Check sheet for the modelled part. Datum: model origin and axes. Units: mm. A direction names the side the tool comes from. Coordinates: 2 decimals unless noted, no trailing zeros. Loops run counter-clockwise (first coordinate to the right, second up) from the corner with the lowest first, then second, coordinate; pieces in that order, holes last.
from build123d import *

# Parameters (mm, degrees)
SKETCH1_R               = 3.65
SKETCH1_W               = 26.6
SKETCH1_H               = 32.3
BOSS_EXTRUDE1_DEPTH     = 8
SKETCH2_W               = 3
SKETCH2_H               = 0.7
BOSS_EXTRUDE2_DEPTH     = 1.2
SKETCH3_W               = 3
SKETCH3_H               = 0.7
BOSS_EXTRUDE3_DEPTH     = 1.2
CHAMFER1_SIZE           = 1.2
CUT_EXTRUDE1_DEPTH      = 85.642077968
CUT_EXTRUDE1_DEPTH_BACK = 85.642077968
SKETCH4_W               = 48.801078557
SKETCH4_H               = 1.4
SKETCH4_W_2             = 10.59579159
SKETCH4_W_3             = 46.838011079
BOSS_EXTRUDE4_START     = -5.4
SKETCH5_W               = 13
SKETCH5_H               = 1.2
SKETCH5_W_2             = 1.2
SKETCH5_H_2             = 13
BOSS_EXTRUDE4_DEPTH     = 2.8
BOSS_EXTRUDE5_REACH     = 77.99
SKETCH7_W               = 1.2
SKETCH7_H               = 1.202104206
SKETCH7_H_2             = 1.201731925
BOSS_EXTRUDE6_DEPTH     = 7
SKETCH8_W               = 1.202104206
SKETCH8_H               = 1.3
SKETCH8_W_2             = 1.201731925
BOSS_EXTRUDE7_DEPTH     = 26.6
SKETCH9_W               = 1.2
SKETCH9_H               = 1.3
BOSS_EXTRUDE8_DEPTH     = 11.797895795


with BuildPart() as part:
    # Sketch1 → Boss-Extrude1 (new body)
    with BuildSketch(Plane(origin=(0, 0, 0), x_dir=(1, 0, 0), z_dir=(0, 1, 0))):
        with BuildLine():
            Line((-7.021942446, 23.451798561), (-15.021942446, 23.451798561))
            Line((-15.021942446, 23.451798561), (-15.021942446, 12.601798561))
            Line((-15.021942446, 12.601798561), (-45.721942446, 10.951798561))
            ThreePointArc((-45.721942446, 10.951798561), (-50.571942446, 6.101798561), (-45.721942446, 1.251798561))
            Line((-45.721942446, 1.251798561), (-15.021942446, -0.398201439))
            Line((-15.021942446, -0.398201439), (-15.021942446, -11.248201439))
            Line((-15.021942446, -11.248201439), (-7.021942446, -11.248201439))
            Line((-7.021942446, -11.248201439), (-5.371942446, -39.098201439))
            ThreePointArc((-5.371942446, -39.098201439), (-0.521942446, -43.948201439), (4.328057554, -39.098201439))
            Line((4.328057554, -39.098201439), (5.978057554, -11.248201439))
            Line((5.978057554, -11.248201439), (13.978057554, -11.248201439))
            Line((13.978057554, -11.248201439), (13.978057554, -0.398201439))
            Line((13.978057554, -0.398201439), (44.678057554, 1.251798561))
            ThreePointArc((44.678057554, 1.251798561), (49.528057554, 6.101798561), (44.678057554, 10.951798561))
            Line((44.678057554, 10.951798561), (13.978057554, 12.601798561))
            Line((13.978057554, 12.601798561), (13.978057554, 23.451798561))
            Line((13.978057554, 23.451798561), (5.978057554, 23.451798561))
            Line((5.978057554, 23.451798561), (4.328057554, 51.301798561))
            ThreePointArc((4.328057554, 51.301798561), (-0.521942446, 56.151798561), (-5.371942446, 51.301798561))
            Line((-5.371942446, 51.301798561), (-7.021942446, 23.451798561))
        make_face()
        with Locations(Location((-0.521942446, -39.098201439, 0), (0, 0, 270))):
            Circle(SKETCH1_R, mode=Mode.SUBTRACT)
        with BuildLine():
            Line((4.775953349, -11.248201439), (3.302651218, -36.115755579))
            ThreePointArc((3.302651218, -36.115755579), (-0.521942446, -34.248201439), (-4.34653611, -36.115755579))
            Line((-4.34653611, -36.115755579), (-5.819838241, -11.248201439))
            Line((-5.819838241, -11.248201439), (4.775953349, -11.248201439))
        make_face(mode=Mode.SUBTRACT)
        with Locations(Location((-45.721942446, 6.101798561, 0), (0, 0, 270))):
            Circle(SKETCH1_R, mode=Mode.SUBTRACT)
        with BuildLine():
            Line((-42.720356894, 9.911389638), (-15.021942446, 11.400066636))
            Line((-15.021942446, 11.400066636), (-15.021942446, 0.803530486))
            Line((-15.021942446, 0.803530486), (-42.720356894, 2.292207484))
            ThreePointArc((-42.720356894, 2.292207484), (-40.871942446, 6.101798561), (-42.720356894, 9.911389638))
        make_face(mode=Mode.SUBTRACT)
        with Locations((-0.521942446, 6.101798561)):
            Rectangle(SKETCH1_W, SKETCH1_H, mode=Mode.SUBTRACT)
        with BuildLine():
            Line((-5.819838241, 23.451798561), (-4.34653611, 48.319352702))
            ThreePointArc((-4.34653611, 48.319352702), (-0.521942446, 46.451798561), (3.302651218, 48.319352702))
            Line((3.302651218, 48.319352702), (4.775953349, 23.451798561))
            Line((4.775953349, 23.451798561), (-5.819838241, 23.451798561))
        make_face(mode=Mode.SUBTRACT)
        with Locations(Location((-0.521942446, 51.301798561, 0), (0, 0, 270))):
            Circle(SKETCH1_R, mode=Mode.SUBTRACT)
        with BuildLine():
            Line((41.676472002, 2.292207484), (13.978057554, 0.803530486))
            Line((13.978057554, 0.803530486), (13.978057554, 11.400066636))
            Line((13.978057554, 11.400066636), (41.676472002, 9.911389638))
            ThreePointArc((41.676472002, 9.911389638), (39.828057554, 6.101798561), (41.676472002, 2.292207484))
        make_face(mode=Mode.SUBTRACT)
        with Locations(Location((44.678057554, 6.101798561, 0), (0, 0, 270))):
            Circle(SKETCH1_R, mode=Mode.SUBTRACT)
    extrude(amount=BOSS_EXTRUDE1_DEPTH)

    # Sketch2 → Boss-Extrude2 (add)
    with BuildSketch(Plane.XY.offset(-22.251798561)):
        with Locations((-2.021942446, 6.05)):
            Rectangle(SKETCH2_W, SKETCH2_H)
        with Locations((0.978057554, 6.05)):
            Rectangle(SKETCH2_W, SKETCH2_H)
    extrude(amount=BOSS_EXTRUDE2_DEPTH)

    # Sketch3 → Boss-Extrude3 (add)
    with BuildSketch(Plane(origin=(0, 0, 10.048201439), x_dir=(-1, 0, 0), z_dir=(0, 0, -1))):
        with Locations((-0.978057554, 6.05)):
            Rectangle(SKETCH3_W, SKETCH3_H)
        with Locations((2.021942446, 6.05)):
            Rectangle(SKETCH3_W, SKETCH3_H)
    extrude(amount=BOSS_EXTRUDE3_DEPTH)

    # Chamfer1
    chamfer1_edges = [part.edges().sort_by_distance(p)[0] for p in [
        (-0.521942446, 5.7, -22.251798561),
        (-0.521942446, 5.7, 10.048201439),
    ]]
    chamfer(chamfer1_edges, length=CHAMFER1_SIZE - 0.0001)  # a hair under: the kernel refuses the full size

    # Sketch4 → Cut-Extrude1 (cut, two sides: drawn at the far end of the back side and taken through both)
    with BuildSketch(Plane(origin=(0, 0, -23.451798561), x_dir=(-1, 0, 0), z_dir=(0, 0, -1)).offset(-CUT_EXTRUDE1_DEPTH_BACK)):
        with Locations((-29.176492628, 3.3)):
            Rectangle(SKETCH4_W, SKETCH4_H)
        with Locations((-29.176492628, 4.7)):
            Rectangle(SKETCH4_W, SKETCH4_H)
        with Locations((0.521942446, 4.7)):
            Rectangle(SKETCH4_W_2, SKETCH4_H)
        with Locations((0.521942446, 3.3)):
            Rectangle(SKETCH4_W_2, SKETCH4_H)
        with Locations((29.238843781, 3.3)):
            Rectangle(SKETCH4_W_3, SKETCH4_H)
        with Locations((29.238843781, 4.7)):
            Rectangle(SKETCH4_W_3, SKETCH4_H)
    extrude(amount=CUT_EXTRUDE1_DEPTH + CUT_EXTRUDE1_DEPTH_BACK, mode=Mode.SUBTRACT)


with BuildPart() as cut_extrude1_piece_1:
    # of the separate pieces the step leaves, piece 1, a body of its own (cut_extrude1_pieces)
    add(part.part.solids().sort_by_distance((-3.521942446, 6.4, 10.048201439))[0])



with BuildPart() as cut_extrude1_piece_2:
    # of the separate pieces the step leaves, piece 2, a body of its own (cut_extrude1_pieces)
    add(part.part.solids().sort_by_distance((12.778057554, 2.6, 10.048201439))[0])


with BuildPart() as cut_extrude1_piece_1_1:
    add(cut_extrude1_piece_1.part)

    add(cut_extrude1_piece_2.part)  # Boss-Extrude4 merges Cut-Extrude1 piece 2
    # Sketch5 → Boss-Extrude4 (add)
    with BuildSketch(Plane(origin=(0, 8, 0), x_dir=(1, 0, 0), z_dir=(0, 1, 0)).offset(BOSS_EXTRUDE4_START)):
        with Locations((-0.521942446, 22.851798561)):
            Rectangle(SKETCH5_W, SKETCH5_H)
        with Locations((-0.521942446, -10.648201439)):
            Rectangle(SKETCH5_W, SKETCH5_H)
        with Locations((-14.421942446, 6.101798561)):
            Rectangle(SKETCH5_W_2, SKETCH5_H_2)
        with Locations((13.378057554, 6.101798561)):
            Rectangle(SKETCH5_W_2, SKETCH5_H_2)
    extrude(amount=BOSS_EXTRUDE4_DEPTH)

    # Sketch6 → Boss-Extrude5 (add, up to next)
    with BuildSketch(Plane(origin=(0, 8, 0), x_dir=(1, 0, 0), z_dir=(0, 1, 0)), mode=Mode.PRIVATE) as boss_extrude5_sk1:
        with BuildLine():
            Line((-5.371942446, 51.301798561), (-4.171942446, 51.301798561))
            ThreePointArc((-4.171942446, 51.301798561), (-0.521942446, 54.951798561), (3.128057554, 51.301798561))
            Line((3.128057554, 51.301798561), (4.328057554, 51.301798561))
            ThreePointArc((4.328057554, 51.301798561), (-0.521942446, 56.151798561), (-5.371942446, 51.301798561))
        make_face()
    boss_extrude5_tool1 = extrude(boss_extrude5_sk1.sketch, amount=-BOSS_EXTRUDE5_REACH, mode=Mode.PRIVATE) - cut_extrude1_piece_1_1.part
    # Sketch6 → Boss-Extrude5 (add, up to next)
    with BuildSketch(Plane(origin=(0, 8, 0), x_dir=(1, 0, 0), z_dir=(0, 1, 0)), mode=Mode.PRIVATE) as boss_extrude5_sk2:
        with BuildLine():
            Line((3.128057554, -39.098201439), (4.328057554, -39.098201439))
            ThreePointArc((4.328057554, -39.098201439), (-0.521942446, -43.948201439), (-5.371942446, -39.098201439))
            Line((-5.371942446, -39.098201439), (-4.171942446, -39.098201439))
            ThreePointArc((-4.171942446, -39.098201439), (-0.521942446, -42.748201439), (3.128057554, -39.098201439))
        make_face()
    boss_extrude5_tool2 = extrude(boss_extrude5_sk2.sketch, amount=-BOSS_EXTRUDE5_REACH, mode=Mode.PRIVATE) - cut_extrude1_piece_1_1.part
    # Sketch6 → Boss-Extrude5 (add, up to next)
    with BuildSketch(Plane(origin=(0, 8, 0), x_dir=(1, 0, 0), z_dir=(0, 1, 0)), mode=Mode.PRIVATE) as boss_extrude5_sk3:
        with BuildLine():
            Line((44.678057554, 9.751798561), (44.678057554, 10.951798561))
            ThreePointArc((44.678057554, 10.951798561), (49.528057554, 6.101798561), (44.678057554, 1.251798561))
            Line((44.678057554, 1.251798561), (44.678057554, 2.451798561))
            ThreePointArc((44.678057554, 2.451798561), (48.328057554, 6.101798561), (44.678057554, 9.751798561))
        make_face()
    boss_extrude5_tool3 = extrude(boss_extrude5_sk3.sketch, amount=-BOSS_EXTRUDE5_REACH, mode=Mode.PRIVATE) - cut_extrude1_piece_1_1.part
    # Sketch6 → Boss-Extrude5 (add, up to next)
    with BuildSketch(Plane(origin=(0, 8, 0), x_dir=(1, 0, 0), z_dir=(0, 1, 0)), mode=Mode.PRIVATE) as boss_extrude5_sk4:
        with BuildLine():
            Line((-45.721942446, 1.251798561), (-45.721942446, 2.451798561))
            ThreePointArc((-45.721942446, 2.451798561), (-49.371942446, 6.101798561), (-45.721942446, 9.751798561))
            Line((-45.721942446, 9.751798561), (-45.721942446, 10.951798561))
            ThreePointArc((-45.721942446, 10.951798561), (-50.571942446, 6.101798561), (-45.721942446, 1.251798561))
        make_face()
    boss_extrude5_tool4 = extrude(boss_extrude5_sk4.sketch, amount=-BOSS_EXTRUDE5_REACH, mode=Mode.PRIVATE) - cut_extrude1_piece_1_1.part
    add(boss_extrude5_tool1.solids().sort_by_distance((-4.771942, 8, -51.410248))[0])
    add(boss_extrude5_tool2.solids().sort_by_distance((-0.521942, 8, 43.839752))[0])
    add(boss_extrude5_tool3.solids().sort_by_distance((44.786507, 8, -10.351799))[0])
    add(boss_extrude5_tool4.solids().sort_by_distance((-45.830392, 8, -10.351799))[0])

    # Sketch7 → Boss-Extrude6 (add)
    with BuildSketch(Plane.XZ):
        with Locations((-14.421942446, -0.202850664)):
            Rectangle(SKETCH7_W, SKETCH7_H)
        with Locations((-14.421942446, -12.000932599)):
            Rectangle(SKETCH7_W, SKETCH7_H_2)
        with Locations((13.378057554, -0.202850664)):
            Rectangle(SKETCH7_W, SKETCH7_H)
        with Locations((13.378057554, -12.000932599)):
            Rectangle(SKETCH7_W, SKETCH7_H_2)
    extrude(amount=BOSS_EXTRUDE6_DEPTH)

    # Sketch8 → Boss-Extrude7 (add)
    with BuildSketch(Plane(origin=(-13.821942446, 0, 0), x_dir=(0, 0, -1), z_dir=(1, 0, 0))):
        with Locations((0.202850664, -6.35)):
            Rectangle(SKETCH8_W, SKETCH8_H)
        with Locations((12.000932599, -6.35)):
            Rectangle(SKETCH8_W_2, SKETCH8_H)
    extrude(amount=BOSS_EXTRUDE7_DEPTH)

    # Sketch9 → Boss-Extrude8 (add)
    with BuildSketch(Plane(origin=(0, 0, -12.601798561), x_dir=(-1, 0, 0), z_dir=(0, 0, -1))):
        with Locations((-13.378057554, -6.35)):
            Rectangle(SKETCH9_W, SKETCH9_H)
        with Locations((14.421942446, -6.35)):
            Rectangle(SKETCH9_W, SKETCH9_H)
    extrude(amount=-BOSS_EXTRUDE8_DEPTH)


solid = cut_extrude1_piece_1_1.part
(1) Draft check along Z on faces 4 (the face through (-14, 5.4, -20)), 5 (the face through (4.05, 1.28, 23.51)), 6 (the face through (29.113, 6.682, -0.415)). Enter one of: pulls with the +Z half, pulls with the -Z half, needs draft (parallel to the pull), parting line crosses it, or undercut.
(2) Section check C-C, the plane y = -3. Enter the section's corners in (x, z).
(3) Section check B-B, the plane y = 4.25. Count the separate pieces of the cut face and the enclosed holes in it, plus the area to 3 significant figures.
(4) Gauge pin test, flat ends, axial feed: P1, Ø4, axis at y = 0, z = -29.5, coming from the +X side; P2, Ø1.3, axis at x = -14.5, y = 4.5, coming from the -Z side; P3, Ø1.3, axis at x = -5.5, z = -0.5, coming from the +Y side; P4, Ø3, axis at y = -2, z = 31, coming from the -X side. Record the tip position at first contact, or that the pin passes through.
(5) Scan lines: line 1 along X through (y, z) = (5.75, -22); line 2 along Z through (x, y) = (40.5, 6.25); line 3 along Y through (x, z) = (-5, -42). Record each from-to range of solid material in increasing order.
(6) Set-up check for faces 1 (the face through (30, 5.4, -1)), 2 (the face through (13, 5.4, -20)), 3 (the face through (10, 7, 11.248)): record each of +Z, -Z, +X, -X, +Y, -Y from which the full face is reachable in a straight line by a thin tool's end or side.
(7) Section check A-A, the plane z = -18. Enter the section's corners in (x, y), plus the area to 3 significant figures.
Determined:
1. face 4: needs draft
1. face 5: undercut
1. face 6: pulls with the +Z half
2. outline: (-15.02, -12.6) - (-13.82, -12.6) - (-13.82, -11.4) - (-15.02, -11.4) - close; (-15.02, -0.8) - (-13.82, -0.8) - (-13.82, 0.4) - (-15.02, 0.4) - close; (12.78, -12.6) - (13.98, -12.6) - (13.98, -11.4) - (12.78, -11.4) - close; (12.78, -0.8) - (13.98, -0.8) - (13.98, 0.4) - (12.78, 0.4) - close
3. separate pieces: 8
3. enclosed holes: 0
3. area: 126 mm2
4. P1: stops at x = 5.74
4. P2: stops at z = -12.6
4. P3: stops at y = -5.7
4. P4: passes through
5. line 1: x = -15.02 to -13.82, -3.52 to 2.48, 12.78 to 13.98
5. line 2: z = -11.18 to -9.97, -8.56 to -3.64, -2.23 to -1.03
5. line 3: y = 0 to 2.6, 5.4 to 8
6. face 1: +Z, -Z
6. face 2: -Z, +X
6. face 3: +Z, +X, +Y, -Y
7. outline: (-15.02, 0) - (-13.82, 0) - (-13.82, 2.6) - (-15.02, 2.6) - close; (-15.02, 5.4) - (-13.82, 5.4) - (-13.82, 8) - (-15.02, 8) - close; (12.78, 0) - (13.98, 0) - (13.98, 2.6) - (12.78, 2.6) - close; (12.78, 5.4) - (13.98, 5.4) - (13.98, 8) - (12.78, 8) - close
7. area: 12.5 mm2
